Read the model definition and answer for the solid it produces. Units are mm, in the model's axes. A direction names the side the tool comes from. Coordinates: 2 decimals unless noted, no trailing zeros. Order: outer loops, then holes, each group sorted by start corner. A loop starts at its lowest first (then second) coordinate and runs counter-clockwise, first axis right, second up.
```python
from build123d import *

# Parameters (mm, degrees)
SKETCH1_W               = 120
SKETCH1_H               = 100
BOSS_EXTRUDE1_DEPTH     = 45
CUT_EXTRUDE1_DEPTH      = 163.55768207
CUT_EXTRUDE1_DEPTH_BACK = 163.55768207
SHELL1_T                = -3


with BuildPart() as part:
    # Sketch1 → Boss-Extrude1 (new body)
    with BuildSketch(Plane(origin=(0, 0, 0), x_dir=(1, 0, 0), z_dir=(0, 1, 0))):
        with Locations((60, 50)):
            Rectangle(SKETCH1_W, SKETCH1_H)
    extrude(amount=BOSS_EXTRUDE1_DEPTH)

    # Sketch2 → Cut-Extrude1 (cut, two sides: drawn at the far end of the back side and taken through both)
    with BuildSketch(Plane(origin=(120, 0, 0), x_dir=(0, 0, -1), z_dir=(1, 0, 0)).offset(-CUT_EXTRUDE1_DEPTH_BACK)):
        Polygon((0, 23), (0, 45), (100, 45), align=None)
    extrude(amount=CUT_EXTRUDE1_DEPTH + CUT_EXTRUDE1_DEPTH_BACK, mode=Mode.SUBTRACT)

    # Shell1
    shell1_openings = [part.faces().sort_by_distance(p)[0] for p in [
        (60, 34, -50),
    ]]
    offset(amount=SHELL1_T, openings=shell1_openings, kind=Kind.INTERSECTION)


solid = part.part
```
1) A flat-ended cylindrical pin translates along its axis: pin 1 Ø1.5 at (x, z) = (17.5, -21.5) entering from +Y. Find the tip coordinate at first contact, or state that the pin passes through.
A:
pin 1: stops at y = 3
2) Which of the six approach directions +Z, -Z, +X, -X, +Y, -Y give full straight-line access (tool end or side, diameter ignored) to faces 1 (the flat face through (59.72, 44.644, -98.381)), 2 (the flat face through (59, 3, -51))?
A:
face 1: +Z, +X, -X, +Y
face 2: +Y
3) Straight lines are drawn through the part: line 1 (Z direction, x = 54, y = 18); line 2 (X direction, y = 15, z = -79); line 3 (Y direction, x = 57.5, z = -48). For each, find the intervals that lie inside material, in ascending order.
A:
line 1: z = -100 to -97, -3 to 0
line 2: x = 0 to 3, 117 to 120
line 3: y = 0 to 3
4) Determine the mould class of faces 3 (the flat face through (59, 0, -51)), 4 (the flat face through (59, 11, 0)), 5 (the flat face through (117, 19, -49)), 6 (the flat face through (3, 19, -49)) for opening direction Z: pulls with the +Z half, pulls with the -Z half, needs draft (parallel to the pull), parting line crosses it, or undercut.
A:
face 3: needs draft
face 4: pulls with the +Z half
face 5: undercut
face 6: undercut
5) A cutting plane is placed at B-B, the plane z = -28.5. Determine the outline of the cut face in (x, y), and give its area (3 significant figures).
A:
outline: (0, 0) - (120, 0) - (120, 29.27) - (117, 29.27) - (117, 3) - (3, 3) - (3, 29.27) - (0, 29.27) - close
area: 518 mm2
6) A cutting plane is placed at A-A, the plane y = 8.5. Determine the outline of the cut face in (x, z).
A:
outline: (0, -100) - (120, -100) - (120, 0) - (0, 0) - close; hole (3, -97) - (117, -97) - (117, -3) - (3, -3) - close
7) A cutting plane is placed at C-C, the plane x = 104.5. Determine the outline of the cut face in (y, z), and give its area (3 significant figures).
A:
outline: (0, -100) - (45, -100) - (44.34, -97) - (3, -97) - (3, -3) - (23.66, -3) - (23, 0) - (0, 0) - close
area: 486 mm2
